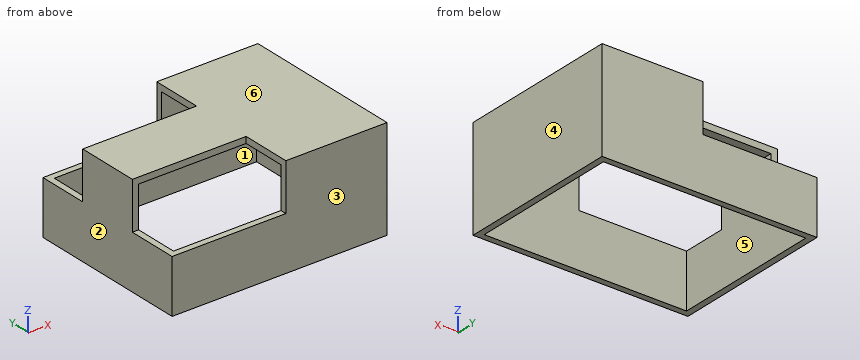
from build123d import *

# Parameters (mm, degrees)
SKETCH1_W           = 86.36
SKETCH1_H           = 66.04
BOSS_EXTRUDE1_DEPTH = 40.64
SKETCH2_W           = 81.28
SKETCH2_H           = 60.96
CUT_EXTRUDE1_DEPTH  = 38.1
SKETCH3_W           = 45.72
SKETCH3_H           = 20.32
CUT_EXTRUDE2_DEPTH  = 19.05
SKETCH4_W           = 45.72
SKETCH4_H           = 20.32
CUT_EXTRUDE3_DEPTH  = 19.05


with BuildPart() as part:
    # Sketch1 → Boss-Extrude1 (new body)
    with BuildSketch(Plane.XY):
        Rectangle(SKETCH1_W, SKETCH1_H)
    extrude(amount=BOSS_EXTRUDE1_DEPTH)

    # Sketch2 → Cut-Extrude1 (cut)
    with BuildSketch(Plane(origin=(0, 0, 0), x_dir=(-1, 0, 0), z_dir=(0, 0, -1))):
        Rectangle(SKETCH2_W, SKETCH2_H)
    extrude(amount=-CUT_EXTRUDE1_DEPTH, mode=Mode.SUBTRACT)

    # Sketch3 → Cut-Extrude2 (cut)
    with BuildSketch(Plane.XY.offset(40.64)):
        with Locations((-20.32, 22.86)):
            Rectangle(SKETCH3_W, SKETCH3_H)
    extrude(amount=-CUT_EXTRUDE2_DEPTH, mode=Mode.SUBTRACT)

    # Sketch4 → Cut-Extrude3 (cut)
    with BuildSketch(Plane.XY.offset(40.64)):
        with Locations((-20.32, -22.86)):
            Rectangle(SKETCH4_W, SKETCH4_H)
    extrude(amount=-CUT_EXTRUDE3_DEPTH, mode=Mode.SUBTRACT)


solid = part.part
Geometry: final body of the model. Coordinates: model frame, mm. Face numbers are marked on the shaded views. A direction names the side the tool comes from. Give positions to 0.01 mm unless a question says otherwise; leave off trailing zeros. Loops run counter-clockwise (first coordinate to the right, second up) from the corner with the lowest first, then second, coordinate; pieces in that order, holes last. Notation, with made-up numbers: M 62.5,-25.75 L 95.5,-25.75 A18 ccw 95.5,-13.75 Z; hole C -26,42.5 d1. An arc over 180 degrees is marked long. Put each result on its own line as item: value.
1) Reachability of the marked faces 5 and 6 from +Z, -Z, +X, -X, +Y, -Y: full face, straight path, thin tool, end or side. Return the list, or none.
Computed values:
face 5: -Z
face 6: +Z, +X, -X, +Y, -Y
2) Cut plane C-C, the plane z = 3.5. Return the cut outline in (x, y).
Computed values:
outline: M -43.18,-33.02 L 43.18,-33.02 L 43.18,33.02 L -43.18,33.02 Z; hole M -40.64,-30.48 L 40.64,-30.48 L 40.64,30.48 L -40.64,30.48 Z
3) Material intervals for L1, parallel to X at y = 11, z = 37.5; L2, parallel to Y at x = 38, z = 14.5; L3, parallel to Z at x = -29, y = -7, sorted ascending. Write a range as from..to.
Computed values:
L1: x = -43.18..-40.64, 40.64..43.18
L2: y = -33.02..-30.48, 30.48..33.02
L3: z = 38.1..40.64
4) First-contact query: P1, Ø15, axis at x = -29.5, z = 33.5, coming from the +Y side; P2, Ø10, axis at x = 8, y = 13.5, coming from the -Z side; P3, Ø12, axis at x = -29, y = -13.5, coming from the +Z side; P4, Ø6, axis at x = -26.5, y = 18, coming from the +Z side. Flat tips, straight axial feed; report the tip coordinate or a pass-through.
Computed values:
P1: stops at y = 12.7
P2: stops at z = 38.1
P3: stops at z = 40.64
P4: passes through
5) Cut plane A-A, the plane y = -16. Return the cut outline in (x, z), plus the area to 3 significant figures.
Computed values:
outline: M -43.18,0 L -40.64,0 L -40.64,21.59 L -43.18,21.59 Z; M 2.54,38.1 L 40.64,38.1 L 40.64,0 L 43.18,0 L 43.18,40.64 L 2.54,40.64 Z
area: 255 mm^2
6) Cut plane B-B, the plane x = -14. Return the cut outline in (y, z), plus the area to 3 significant figures.
Computed values:
outline: M -33.02,0 L -30.48,0 L -30.48,21.59 L -33.02,21.59 Z; M -12.7,38.1 L 12.7,38.1 L 12.7,40.64 L -12.7,40.64 Z; M 30.48,0 L 33.02,0 L 33.02,21.59 L 30.48,21.59 Z
area: 174 mm^2
7) Cut plane D-D, the plane z = 31. Return the cut outline in (x, y), plus the area to 3 significant figures.
Computed values:
outline: M -43.18,-12.7 L -40.64,-12.7 L -40.64,12.7 L -43.18,12.7 Z; M 2.54,-33.02 L 43.18,-33.02 L 43.18,33.02 L 2.54,33.02 L 2.54,30.48 L 40.64,30.48 L 40.64,-30.48 L 2.54,-30.48 Z
area: 426 mm^2
8) Mould query, pull axis X, two halves, no side actions, for the marked faces 1, 2, 3 and 4. Classes: released by +X, released by -X, zero draft, split by the parting line, or undercut.
Computed values:
face 1: undercut
face 2: released by -X
face 3: zero draft
face 4: released by +X
